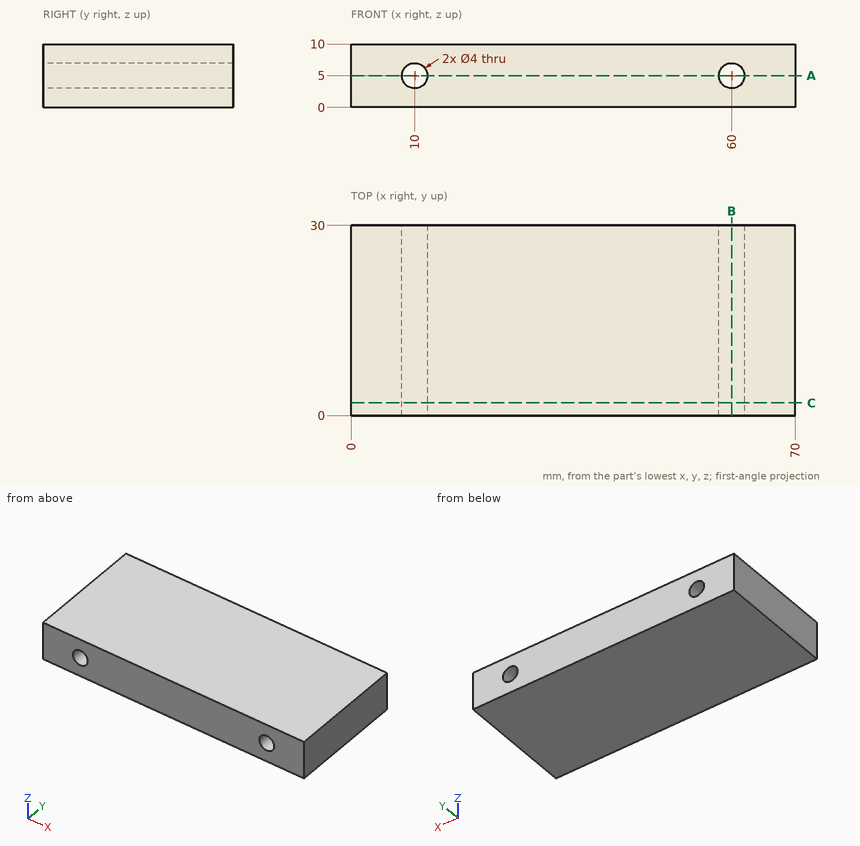
Answer from the drawing. Dimensions are ordinates in mm from the lowest x, y and z of the part. Coordinates: 2 decimals unless noted, no trailing zeros. Write each loop counter-clockwise with the first axis right and the second up, starting at its lowest first coordinate (ties: lowest second). Pieces come first, ordered by that corner, then holes. Notation, with made-up numbers: (39, 44.25) - (89, 44.25) arc R7 ccw to (89, 48.25) - close; hole circle Ø10 at (-38, 65.5). An arc over 180 degrees is marked (long way). Return JSON: item names as keys, results as strings.
1. The part is cut by section A-A on z = 5. Determine the outline of the cut face in (x, y).
Final values:
{"outline": "(0, 0) - (8, 0) - (8, 30) - (0, 30) - close; (12, 0) - (58, 0) - (58, 30) - (12, 30) - close; (62, 0) - (70, 0) - (70, 30) - (62, 30) - close"}
2. The part is cut by section C-C on y = 2. Determine the outline of the cut face in (x, z).
Final values:
{"outline": "(0, 0) - (70, 0) - (70, 10) - (0, 10) - close; hole circle Ø4 at (10, 5); hole circle Ø4 at (60, 5)"}
3. The part is cut by section B-B on x = 60. Determine the outline of the cut face in (y, z), then the cut area to 3 significant figures.
Final values:
{"outline": "(0, 0) - (30, 0) - (30, 3) - (0, 3) - close; (0, 7) - (30, 7) - (30, 10) - (0, 10) - close", "area": "180 mm^2"}
4. Consider line 1 along Z through (x, y) = (60, 20); line 2 along X through (y, z) = (18.5, 6.75); line 3 along X through (y, z) = (4.5, 4). Determine where each line is inside the solid, lowest interval first.
Final values:
{"line 1": "0 to 3, 7 to 10", "line 2": "0 to 9.03, 10.97 to 59.03, 60.97 to 70", "line 3": "0 to 8.27, 11.73 to 58.27, 61.73 to 70"}
